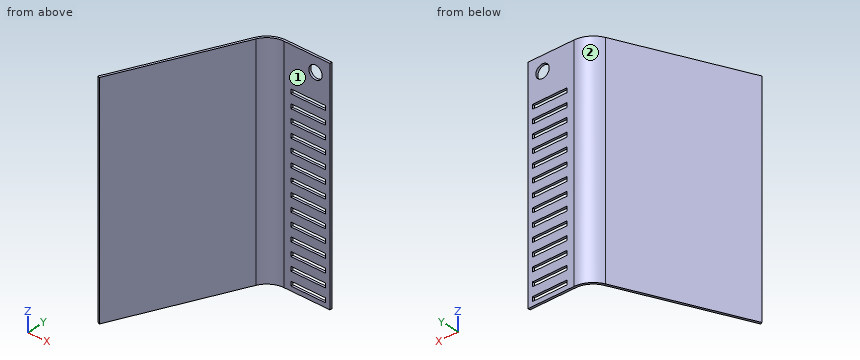
from build123d import *

# Parameters (mm, degrees)
EXTRUDE_THIN1_DEPTH = 500
SKETCH2_W           = 155.95
SKETCH2_H           = 20
CUT_EXTRUDE1_DEPTH  = 590.213534275
LPATTERN1_COUNT     = 14
LPATTERN1_PITCH     = 60
SKETCH3_R           = 30
CUT_EXTRUDE2_DEPTH  = 590.213534275


with BuildPart() as part:
    # Sketch1 → Extrude-Thin1 (new body, symmetric)
    with BuildSketch(Plane.XY):
        with BuildLine():
            Line((0, 0), (-205.95, 0))
            ThreePointArc((-205.95, 0), (-259.885879639, -15.792394123), (-296.786225905, -58.181582248))
            Line((-296.786225905, -58.181582248), (-539.333048865, -585.0316925))
            Line((-539.333048865, -585.0316925), (-530.249426274, -589.213534275))
            Line((-530.249426274, -589.213534275), (-287.702603315, -62.363424024))
            ThreePointArc((-287.702603315, -62.363424024), (-254.492291675, -24.21315471), (-205.95, -10))
            Line((-205.95, -10), (0, -10))
            Line((0, -10), (0, 0))
        make_face()
    extrude(amount=EXTRUDE_THIN1_DEPTH, both=True)

    # Sketch2 → Cut-Extrude1 (cut, through all)
    with BuildSketch(Plane(origin=(0, 0, 0), x_dir=(1, 0, 0), z_dir=(0, 1, 0))):
        with Locations((-97.975, 470)):
            Rectangle(SKETCH2_W, SKETCH2_H)
    cut_extrude1 = extrude(amount=-CUT_EXTRUDE1_DEPTH, mode=Mode.SUBTRACT)

    # LPattern1: Cut-Extrude1 ×14
    with Locations(*[(0, 0, i * LPATTERN1_PITCH) for i in range(1, LPATTERN1_COUNT)]):
        add(cut_extrude1, mode=Mode.SUBTRACT)

    # Sketch3 → Cut-Extrude2 (cut, through all)
    with BuildSketch(Plane(origin=(0, 0, 0), x_dir=(1, 0, 0), z_dir=(0, 1, 0))):
        with Locations((-65, -435)):
            Circle(SKETCH3_R)
    extrude(amount=-CUT_EXTRUDE2_DEPTH, mode=Mode.SUBTRACT)


solid = part.part
CAD build for the part. Positions are in the model's coordinates, mm. Face numbers are marked on the shaded views. A direction names the side the tool comes from. Round coordinates to 2 decimals unless told otherwise and drop trailing zeros. Order: outer loops, then holes, each group sorted by start corner. A loop starts at its lowest first (then second) coordinate and runs counter-clockwise, first axis right, second up. Notation, with made-up numbers: (21.25, 65) -> (32.25, 65) arc R12 cw to (32.25, 73) -> close; hole circle Ø11 at (-20, 77.5). An arc over 180 degrees is marked (long way). Write item = value, one per line. Start each with the question number.
(1) Which spindle directions (+Z, -Z, +X, -X, +Y, -Y) get a long thin tool onto all of the face, cutting with end or side? Do the marked faces 1 and 2. Say none if no direction does.
(2) Cut at B-B, the plane z = -380. List the corners of the cut face in (x, y), then the cut area to 3 significant figures.
(3) Cut at C-C, the plane x = -65. State how many separate pieces and enclosed holes the cut face has, then the cut area to 3 significant figures.
(4) Cut at D-D, the plane y = -144.5. List the corners of the cut face in (x, z).
(5) Pin check, flat tips, straight feed: P1, Ø5, axis at y = -92.5, z = -222.5, coming from the +X side; P2, Ø8, axis at y = -256.5, z = -73.5, coming from the -X side; P3, Ø3, axis at x = -339.5, z = -230, coming from the +Y side. Stop position of each tip, or through.
(6) Cut at A-A, the plane z = 435. List the corners of the cut face in (x, y), then the cut area to 3 significant figures.
(7) Probe line 1 (Y direction, x = -159, z = 288); line 2 (Y direction, x = -415, z = 425); line 3 (X direction, y = -7.75, z = 435). List the from-to ranges inside material, lowest first. Write a range as [from, to].
Model answer:
q1.face_1 = +Z, -Z, +X, -Y
q1.face_2 = +Z, -Z, -X, +Y
q2.outline = (-539.33, -585.03) -> (-530.25, -589.21) -> (-287.7, -62.36) arc R90 cw to (-205.95, -10) -> (0, -10) -> (0, 0) -> (-205.95, 0) arc R100 ccw to (-296.79, -58.18) -> close
q2.area = 8,940 mm2
q3.separate_pieces = 16
q3.enclosed_holes = 0
q3.area = 6,600 mm2
q4.outline = (-336.52, -500) -> (-325.52, -500) -> (-325.52, 500) -> (-336.52, 500) -> close
q5.P1 = -300.43
q5.P2 = -389.93
q5.P3 = -147.7
q6.outline = (-539.33, -585.03) -> (-530.25, -589.21) -> (-287.7, -62.36) arc R90 cw to (-205.95, -10) -> (-95, -10) -> (-95, 0) -> (-205.95, 0) arc R100 ccw to (-296.79, -58.18) -> close; (-35, -10) -> (0, -10) -> (0, 0) -> (-35, 0) -> close
q6.area = 8,340 mm2
q7.line_1 = [-10, 0]
q7.line_2 = [-338.87, -314.96]
q7.line_3 = [-244.55, -95], [-35, 0]
